Source: CAD feature listing. Evaluate the final solid. Frame: model axes, mm. A direction names the side the tool comes from. Round coordinates to 2 decimals unless told otherwise and drop trailing zeros. Loops run counter-clockwise (first coordinate to the right, second up) from the corner with the lowest first, then second, coordinate; pieces in that order, holes last. Notation, with made-up numbers: (56.5, 40.25) -> (113.5, 40.25) arc R24 ccw to (113.5, 65.25) -> close; hole circle Ø2 at (71, -40). An arc over 180 degrees is marked (long way). Write item = value, one per line.
from build123d import *

# Parameters (mm, degrees)
F1_DEPTH    = 6
F2_R        = 12.5
F3_DEPTH    = 6
F5_D        = 15
F6_T1_DEPTH = 6
F6_T3_DEPTH = 46
F7_R        = 5


# Not quite as in the source:
# - a fillet or chamfer that OpenCascade refuses, or shapes differently, is made with other operations: its cross-section is extruded or revolved along the edge and cut away or added


with BuildPart() as f1:
    # F0 (on Front) → F1 (new body)
    with BuildSketch(Plane.XZ):
        Polygon((0, 0), (0, 40), (-25, 40), (-25, 24), (-19, 24), (-19, 34), (-6, 34), (-6, 0), align=None)
    extrude(amount=F1_DEPTH)

    # F2 (on Front) → F3 (join)
    with BuildSketch(Plane.XZ):
        with Locations((0, -10)):
            Circle(F2_R)
    extrude(amount=F3_DEPTH)

    # F5 (through all)
    with Locations(Plane.XZ.offset(6)):
        with Locations((0, -10)):
            Hole(F5_D / 2)

    # F6: fillet of radius 8 on 4 edges, made by hand

    # F6_s2 → F6_t1 (join)
    with BuildSketch(Plane.XZ):
        with BuildLine():
            ThreePointArc((-6, 26), (-8.3431457505, 31.6568542495), (-14, 34))
            Line((-14, 34), (-6, 34))
            Line((-6, 34), (-6, 26))
        make_face()
        with BuildLine():
            ThreePointArc((-11, 34), (-16.6568542495, 31.6568542495), (-19, 26))
            Line((-19, 26), (-19, 34))
            Line((-19, 34), (-11, 34))
        make_face()
    extrude(amount=F6_T1_DEPTH)

    # F6_s4 → F6_t3 (cut)
    with BuildSketch(Plane.XZ.offset(-20)):
        with BuildLine():
            ThreePointArc((0, 32), (-2.3431457505, 37.6568542495), (-8, 40))
            Line((-8, 40), (0, 40))
            Line((0, 40), (0, 32))
        make_face()
        with BuildLine():
            ThreePointArc((-17, 40), (-22.6568542495, 37.6568542495), (-25, 32))
            Line((-25, 32), (-25, 40))
            Line((-25, 40), (-17, 40))
        make_face()
    extrude(amount=F6_T3_DEPTH, mode=Mode.SUBTRACT)

    # F7
    f7_edges = [f1.edges().sort_by_distance(p)[0] for p in [
        (-6, -3, 0.965856),
        (0, -3, 2.5),
    ]]
    fillet(f7_edges, radius=F7_R)


solid = f1.part
1. Line query: probe 1 along X at (y, z) = (-3.7, 26); probe 2 along X at (y, z) = (-1.05, 32); probe 3 along X at (y, z) = (-0.8, 17.5). Output: solid intervals per line, ascending. Write a range as from..to.
Evaluation:
probe_1 = -25..-19, -6..0
probe_2 = -25..-16.29, -8.71..0
probe_3 = -6..0
2. Section query A-A (z = -10). Return the cut outline in (x, y).
Evaluation:
outline = (-12.5, -6) -> (-7.5, -6) -> (-7.5, 0) -> (-12.5, 0) -> close; (7.5, -6) -> (12.5, -6) -> (12.5, 0) -> (7.5, 0) -> close
3. Set-up query: faces 1 (the face through (-6.475, -2.958, 1.484)), 2 (the face through (-19, -3, 25)), 3 (the face through (-22, -3, 24)). Return all of +Z, -Z, +X, -X, +Y, -Y with unobstructed straight access to the full face (end or side cutting, diameter ignored); none if empty.
Evaluation:
face_1 = -X, +Y, -Y
face_2 = -Z, +Y, -Y
face_3 = -Z, -X, +Y, -Y
4. Section query D-D (z = 12). Return the cut outline in (x, y), then the cut area to 3 significant figures.
Evaluation:
outline = (-6, -6) -> (0, -6) -> (0, 0) -> (-6, 0) -> close
area = 36.0 mm²
5. Section query B-B (y = -4.65). Return the cut outline in (x, z).
Evaluation:
outline = (-25, 24) -> (-19, 24) -> (-19, 26) arc R8 cw to (-12.5, 33.86) arc R8 cw to (-6, 26) -> (-6, 3.61) arc R5 cw to (-7.86, -0.28) arc R12.5 ccw (long way) to (3.57, 1.98) arc R5 cw to (0, 6.77) -> (0, 32) arc R8 ccw to (-8, 40) -> (-17, 40) arc R8 ccw to (-25, 32) -> close; hole circle Ø15 at (0, -10)
6. Mould query, pull axis Z, two halves, no side actions, for faces 4 (the face through (-12, -3, 40)), 5 (the face through (-7.787, -2.958, 31.039)), 6 (the face through (-6, -3, 15)), 7 (the face through (-3, -6, 11)). Classes: released by +Z, released by -Z, zero draft, split by the parting line, or undercut.
Evaluation:
face_4 = released by +Z
face_5 = undercut
face_6 = undercut
face_7 = zero draft
7. Section query C-C (x = -4.5). Return the cut outline in (y, z), then the cut area to 3 significant figures.
Evaluation:
outline = (-6, -21.66) -> (0, -21.66) -> (0, -16) -> (-6, -16) -> close; (-6, -4) -> (0, -4) -> (0, 39.19) -> (-6, 39.19) -> close
area = 293 mm²
8. Contact query for flat-ended pins moving along their axis: pin 1 Ø3 at (x, y) = (-4, -2) entering from +Z; pin 2 Ø1 at (x, y) = (-4, -5) entering from -Z; pin 3 Ø2 at (y, z) = (-2.5, 24.5) entering from +X. Output: stop coordinate, or through.
Evaluation:
pin_1 = 39.6
pin_2 = -22
pin_3 = 0
